Geometry check sheet. Reference: drawing and pictorial views, mm from the part's lowest x, y, z. A direction names the side the tool comes from. Round coordinates to 2 decimals unless told otherwise and drop trailing zeros. Write each loop counter-clockwise with the first axis right and the second up, starting at its lowest first coordinate (ties: lowest second). Pieces come first, ordered by that corner, then holes. Notation, with made-up numbers: (22.5, 77.25) - (54.5, 77.25) arc R4 ccw to (54.5, 81.25) - close; hole circle Ø1 at (-8.75, -20.75). An arc over 180 degrees is marked (long way). Return JSON: item names as keys, results as strings.
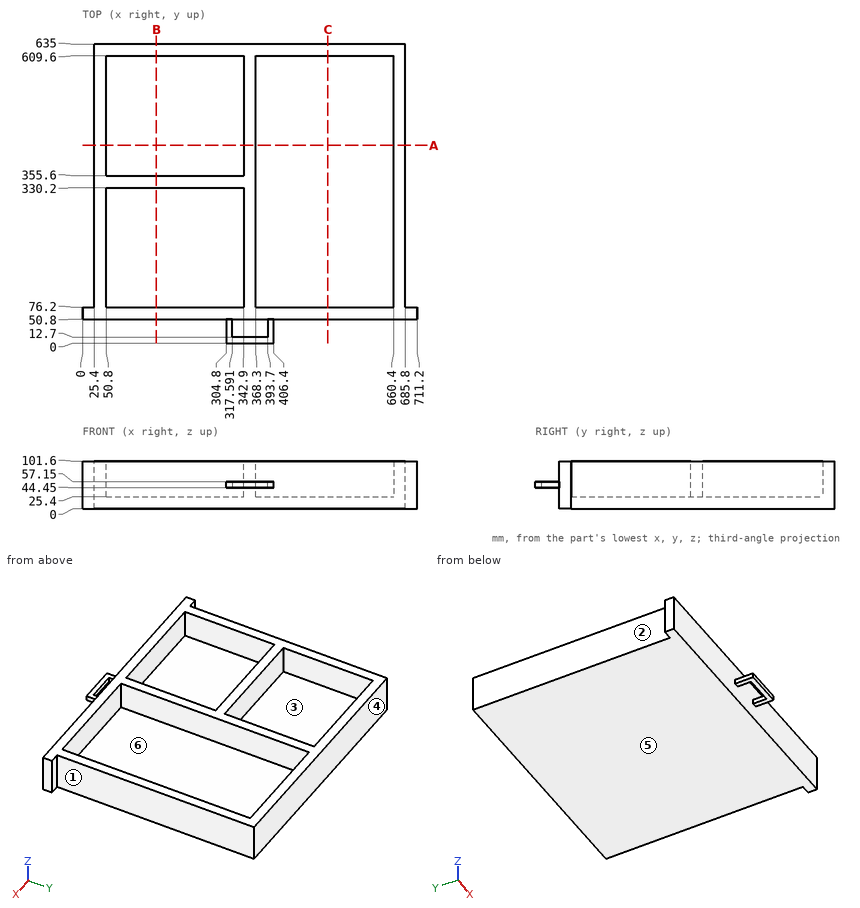
(1) Material ranges on line 1 along Y through (x, z) = (244.5, 43); line 2 along X through (y, z) = (554.5, 70); line 3 along Y through (x, z) = (327, 47.5), recorded low to high. Write a range as [from, to].
Response values:
{"line 1": "y = [50.8, 76.2], [330.2, 355.6], [609.6, 635]", "line 2": "x = [25.4, 50.8], [342.9, 368.3], [660.4, 685.8]", "line 3": "y = [0, 12.7], [50.8, 76.2], [330.2, 355.6], [609.6, 635]"}
(2) Release check for a two-part mould opening along Y. For the marked faces 4, 5 and 6 record: pulls with the +Y half, pulls with the -Y half, needs draft (parallel to the pull), parting line crosses it, or undercut.
Response values:
{"face 4": "pulls with the +Y half", "face 5": "needs draft", "face 6": "undercut"}
(3) Section check B-B, the plane x = 157. Enter the section's corners in (y, z).
Response values:
{"outline": "(50.8, 0) - (635, 0) - (635, 101.6) - (609.6, 101.6) - (609.6, 25.4) - (355.6, 25.4) - (355.6, 101.6) - (330.2, 101.6) - (330.2, 25.4) - (76.2, 25.4) - (76.2, 101.6) - (50.8, 101.6) - close"}
(4) Section check C-C, the plane x = 521. Enter the section's corners in (y, z).
Response values:
{"outline": "(50.8, 0) - (635, 0) - (635, 101.6) - (609.6, 101.6) - (609.6, 25.4) - (76.2, 25.4) - (76.2, 101.6) - (50.8, 101.6) - close"}
(5) Gauge pin test, flat ends, axial feed: pin 1 (12 mm diameter, centred on x = 557.5, z = 23.5, fed in from -Y); pin 2 (10 mm diameter, centred on y = 30, z = 52.5, fed in from +X); pin 3 (7.5 mm diameter, centred on x = 693.5, z = 53, fed in from +Y); pin 4 (3 mm diameter, centred on x = 106, y = 116.5, fed in from -Z). Record the tip position at first contact, or that the pin passes through.
Response values:
{"pin 1": "stops at y = 50.8", "pin 2": "stops at x = 406.4", "pin 3": "stops at y = 76.2", "pin 4": "stops at z = 0"}
(6) Access from +Z, -Z, +X, -X, +Y, -Y to the whole of each face (thin tool, end or side, straight path). Record for the marked faces 1, 2 and 3.
Response values:
{"face 1": "+Z, -Z, +X, +Y", "face 2": "+Z, -Z, -X, +Y", "face 3": "+Z"}
(7) Section check A-A, the plane y = 420. Enter the section's corners in (x, z).
Response values:
{"outline": "(25.4, 0) - (685.8, 0) - (685.8, 101.6) - (660.4, 101.6) - (660.4, 25.4) - (368.3, 25.4) - (368.3, 101.6) - (342.9, 101.6) - (342.9, 25.4) - (50.8, 25.4) - (50.8, 101.6) - (25.4, 101.6) - close"}
